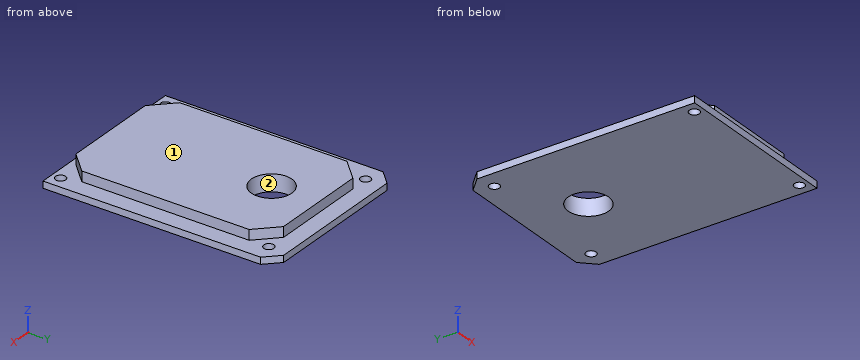
from build123d import *

# Parameters (mm, degrees)
SKETCH1_W           = 51.23
SKETCH1_H           = 68.5
BOSS_EXTRUDE1_DEPTH = 2
CHAMFER1_SIZE       = 4
SKETCH3_W           = 40.93
SKETCH3_H           = 61.5
BOSS_EXTRUDE3_DEPTH = 3
CHAMFER2_SIZE       = 5.95
SKETCH4_R           = 1.5
CUT_EXTRUDE1_DEPTH  = 43.874126522
SKETCH5_R           = 6
CUT_EXTRUDE2_DEPTH  = 44.060314966


with BuildPart() as part:
    # Sketch1 → Boss-Extrude1 (new body)
    with BuildSketch(Plane.XY):
        Rectangle(SKETCH1_W, SKETCH1_H)
    extrude(amount=BOSS_EXTRUDE1_DEPTH)

    # Chamfer1
    chamfer1_edges = [part.edges().sort_by_distance(p)[0] for p in [
        (-25.615, 34.25, 1),
        (25.615, 34.25, 1),
    ]]
    chamfer(chamfer1_edges, length=CHAMFER1_SIZE)

    # Sketch3 → Boss-Extrude3 (add)
    with BuildSketch(Plane.XY.offset(2)):
        with Locations((0, -1.6)):
            Rectangle(SKETCH3_W, SKETCH3_H)
    extrude(amount=BOSS_EXTRUDE3_DEPTH)

    # Chamfer2
    chamfer2_edges = [part.edges().sort_by_distance(p)[0] for p in [
        (20.465, -32.35, 3.5),
        (20.465, 29.15, 3.5),
        (-20.465, 29.15, 3.5),
        (-20.465, -32.35, 3.5),
    ]]
    chamfer(chamfer2_edges, length=CHAMFER2_SIZE)

    # Sketch4 → Cut-Extrude1 (cut, through all)
    with BuildSketch(Plane.XY.offset(2)):
        with Locations((-20.242100654, 28.877100654)):
            Circle(SKETCH4_R)
        with Locations((20.242100654, 28.877100654)):
            Circle(SKETCH4_R)
        with Locations((21.974423525, -31.604966365)):
            Circle(SKETCH4_R)
        with Locations((-21.974423525, -31.604966365)):
            Circle(SKETCH4_R)
    extrude(amount=-CUT_EXTRUDE1_DEPTH, mode=Mode.SUBTRACT)

    # Sketch5 → Cut-Extrude2 (cut, through all)
    with BuildSketch(Plane(origin=(0, 0, 0), x_dir=(-1, 0, 0), z_dir=(0, 0, -1))):
        with Locations((0, 15.35)):
            Circle(SKETCH5_R)
    extrude(amount=-CUT_EXTRUDE2_DEPTH, mode=Mode.SUBTRACT)


solid = part.part
Here's how the part is built. I have some questions about the finished solid (model axes, mm). Face numbers are marked on the shaded views. Give positions to 0.01 mm unless a question says otherwise; leave off trailing zeros. Loops run counter-clockwise (first coordinate to the right, second up) from the corner with the lowest first, then second, coordinate; pieces in that order, holes last. Notation, with made-up numbers: (82, -30) -> (137, -30) arc R6 ccw to (137, -24) -> close; hole circle Ø1 at (50.5, 69). An arc over 180 degrees is marked (long way). One line per item, written item: value.
Q1. Suppose I cut it at D-D on x = -7. Please give me the cut outline in (y, z), then the cut area to 4 significant figures.
Answers follow:
outline: (-34.25, 0) -> (34.25, 0) -> (34.25, 2) -> (29.15, 2) -> (29.15, 5) -> (-32.35, 5) -> (-32.35, 2) -> (-34.25, 2) -> close
area: 321.5 mm^2
Q2. Suppose I cut it at B-B on z = 4.1. Please give me the cut outline in (x, y) (3 decimals), then the cut area to 3 significant figures.
Answers follow:
outline: (-20.465, -26.4) -> (-14.515, -32.35) -> (14.515, -32.35) -> (20.465, -26.4) -> (20.465, 23.2) -> (14.515, 29.15) -> (-14.515, 29.15) -> (-20.465, 23.2) -> close; hole circle Ø12 at (0, 15.35)
area: 2,330 mm^2
Q3. Suppose I cut it at A-A on y = 15.35. Please give me the cut outline in (x, z) (3 decimals).
Answers follow:
outline: (-25.615, 0) -> (-6, 0) -> (-6, 5) -> (-20.465, 5) -> (-20.465, 2) -> (-25.615, 2) -> close; (6, 0) -> (25.615, 0) -> (25.615, 2) -> (20.465, 2) -> (20.465, 5) -> (6, 5) -> close
Q4. I'm going to push flat-ended pins straight in: pin 1 Ø2.5 at (x, y) = (-20.24, 28.88) entering from +Z; pin 2 Ø5 at (x, y) = (21.97, -31.6) entering from +Z; pin 3 Ø2.5 at (y, z) = (-8, 3.5) entering from +X (3 decimals); pin 4 Ø1.5 at (y, z) = (4.5, 3) entering from -X (3 decimals). Where does each tip first touch, or does it pass through?
Answers follow:
pin 1: through
pin 2: z = 2
pin 3: x = 20.465
pin 4: x = -20.465
Q5. Suppose I cut it at C-C on x = 0. Please give me the cut outline in (y, z), then the cut area to 4 significant figures.
Answers follow:
outline: (-34.25, 0) -> (9.35, 0) -> (9.35, 5) -> (-32.35, 5) -> (-32.35, 2) -> (-34.25, 2) -> close; (21.35, 0) -> (34.25, 0) -> (34.25, 2) -> (29.15, 2) -> (29.15, 5) -> (21.35, 5) -> close
area: 261.5 mm^2
Q6. If I drill on line 1 along Y through (x, z) = (13, 2.15); line 2 along X through (y, z) = (15, 0.65) (3 decimals); line 3 along X through (y, z) = (7.5, 3.65) (3 decimals), over which ranges is the centre line in solid material (lowest first)?
Answers follow:
line 1: -32.35 to 29.15
line 2: -25.615 to -5.99, 5.99 to 25.615
line 3: -20.465 to 20.465
Q7. We'd pull the mould along Y, two halves only. Please class the marked faces 1 and 2: pulls with the +Y half, pulls with the -Y half, needs draft (parallel to the pull), parting line crosses it, or undercut.
Answers follow:
face 1: needs draft
face 2: undercut
